Build history of the part. All positions in model axes, mm. Face numbers are marked on the shaded views. A direction names the side the tool comes from. Round coordinates to 2 decimals unless told otherwise and drop trailing zeros. Loops run counter-clockwise (first coordinate to the right, second up) from the corner with the lowest first, then second, coordinate; pieces in that order, holes last. Notation, with made-up numbers: (-26.5, 18.25) -> (19.5, 18.25) arc R33 cw to (19.5, 56.25) -> close; hole circle Ø11 at (-19.75, 26.5). An arc over 180 degrees is marked (long way). Put each result on its own line as item: value. Start each with the question number.
Item 1: Drill centre lines: probe 1 along Y at (x, z) = (67, 1); probe 2 along Z at (x, y) = (21, 14.5); probe 3 along Y at (x, z) = (-8, -48.5). Where is each one in solid material? Low to high. Write a range as [from, to].
Item 2: Flat gauge pins, fed straight in: pin 1 Ø5 at (y, z) = (3, -14.5) entering from +X; pin 2 Ø2 at (x, y) = (67, 36) entering from -Z; pin 3 Ø0.6 at (x, y) = (-4.5, -7.5) entering from -Z; pin 4 Ø4 at (x, z) = (51.5, -25.5) entering from -Y. Where does each tip first touch, or does it go through?
Item 3: Cut at D-D, the plane y = 36. List the corners of the cut face in (x, z), plus the area to 3 significant figures.
Item 4: Cut at C-C, the plane z = -14. List the corners of the cut face in (x, y), plus the area to 3 significant figures.
Item 5: Cut at A-A, the plane y = 0. List the corners of the cut face in (x, z) (3 decimals), plus the area to 3 significant figures.
Item 6: Cut at B-B, the plane x = 67. List the corners of the cut face in (y, z), plus the area to 3 significant figures.
Item 7: Tool access for the marked faces 1 and 2: list every direction of +Z, -Z, +X, -X, +Y, -Y with a clear straight run to the whole face (end or side of a thin tool).
Item 8: Pull direction Z, two halves, no side cores. Call the marked faces 3, 4 and 5: +Z half, -Z half, draft (parallel to the pull), parting line (faces both ways), or undercut.
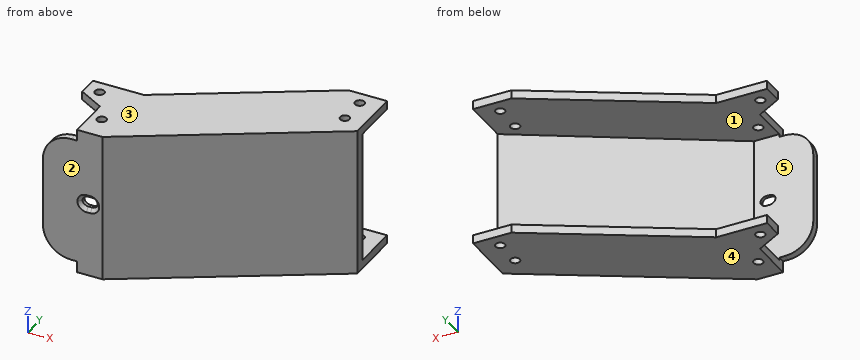
```python
from build123d import *

# Parameters (mm, degrees)
SKETCH1_R                                      = 1.65
BOSS_EXTRUDE1_DEPTH                            = 3
SKETCH1_3_W                                    = 9
SKETCH1_3_H                                    = 2.5
BOSS_EXTRUDE2_DEPTH                            = 46.6
BOSS_EXTRUDE3_START                            = -49.6
SKETCH1_4_R                                    = 1.65
SKETCH1_4_W                                    = 9
SKETCH1_4_H                                    = 2.5
BOSS_EXTRUDE3_DEPTH                            = 3
CUT_EXTRUDE1_DEPTH                             = 88.5
SKETCH3_W                                      = 44.6
SKETCH3_H                                      = 2.5
BOSS_EXTRUDE4_DEPTH                            = 12
FILLET1_R                                      = 10
CSK_START                                      = -9
CSK_SLOT_FOR_M3_COUNTERSUNK_FLAT_HEAD_SC_DEPTH = 3


with BuildPart() as part:
    # Sketch1 → Boss-Extrude1 (new body)
    with BuildSketch(Plane.XY):
        Polygon((-13, 18.856406461), (-13, 11.696152423), (-4, 6.5), (-4, -9), (5, -9), (74, 31), (74, 51), (60.447698856, 51), (5, 18.856406461), align=None)
        Circle(SKETCH1_R, mode=Mode.SUBTRACT)
        with Locations((-8, 13.856406461)):
            Circle(SKETCH1_R, mode=Mode.SUBTRACT)
        with Locations((67, 46)):
            Circle(SKETCH1_R, mode=Mode.SUBTRACT)
        with Locations((67, 36)):
            Circle(SKETCH1_R, mode=Mode.SUBTRACT)
    extrude(amount=BOSS_EXTRUDE1_DEPTH)

    # Sketch1<3> → Boss-Extrude2 (add)
    with BuildSketch(Plane.XY):
        with Locations((0.5, -7.75)):
            Rectangle(SKETCH1_3_W, SKETCH1_3_H)
        Polygon((74, 34.467646849), (5, -6.5), (5, -9), (74, 31), align=None)
    extrude(amount=-BOSS_EXTRUDE2_DEPTH)

    # Sketch1<4> → Boss-Extrude3 (add)
    # profile 1 of 4: a face of its own
    with BuildSketch(Plane.XY.offset(BOSS_EXTRUDE3_START)):
        Polygon((5, 18.856406461), (-13, 18.856406461), (-13, 11.696152423), (-4, 6.5), (-4, -6.5), (5, -6.5), align=None)
        Circle(SKETCH1_4_R, mode=Mode.SUBTRACT)
        with Locations((-8, 13.856406461)):
            Circle(SKETCH1_4_R, mode=Mode.SUBTRACT)
    # profile 2 of 4: a face of its own
    with BuildSketch(Plane.XY.offset(BOSS_EXTRUDE3_START)):
        with Locations((0.5, -7.75)):
            Rectangle(SKETCH1_4_W, SKETCH1_4_H)
    # profile 3 of 4: a face of its own
    with BuildSketch(Plane.XY.offset(BOSS_EXTRUDE3_START)):
        Polygon((74, 34.467646849), (5, -6.5), (5, -9), (74, 31), align=None)
    # profile 4 of 4: a face of its own
    with BuildSketch(Plane.XY.offset(BOSS_EXTRUDE3_START)):
        Polygon((60.447698856, 51), (5, 18.856406461), (5, -6.5), (74, 34.467646849), (74, 51), align=None)
        with Locations((67, 36)):
            Circle(SKETCH1_4_R, mode=Mode.SUBTRACT)
        with Locations((67, 46)):
            Circle(SKETCH1_4_R, mode=Mode.SUBTRACT)
    extrude(amount=BOSS_EXTRUDE3_DEPTH)

    # Sketch2 → Cut-Extrude1 (cut)
    with BuildSketch(Plane.XZ.offset(9)):
        with BuildLine():
            Line((1, -24.95), (-1, -24.95))
            ThreePointArc((-1, -24.95), (-2.65, -23.3), (-1, -21.65))
            Line((-1, -21.65), (1, -21.65))
            ThreePointArc((1, -21.65), (2.65, -23.3), (1, -24.95))
        make_face()
    extrude(amount=-CUT_EXTRUDE1_DEPTH, mode=Mode.SUBTRACT)

    # Sketch3 → Boss-Extrude4 (add)
    with BuildSketch(Plane.ZY.offset(4)):
        with Locations((-23.3, -7.75)):
            Rectangle(SKETCH3_W, SKETCH3_H)
    extrude(amount=BOSS_EXTRUDE4_DEPTH)

    # Fillet1
    fillet1_edges = [part.edges().sort_by_distance(p)[0] for p in [
        (-16, -7.75, -45.6),
        (-16, -7.75, -1),
    ]]
    fillet(fillet1_edges, radius=FILLET1_R)

    # CSK SLOT for M3 Countersunk Flat Head Screw1: read off the stored shape, not the designer's step
    # CSK SLOT for M3 Countersunk Flat Hea 2 → CSK SLOT for M3 Countersunk Flat Head Screw1 (cut)
    with BuildSketch(Plane(origin=(0, 0, 0), x_dir=(1, 0, 0), z_dir=(0, 1, 0)).offset(CSK_START)):
        with BuildLine():
            ThreePointArc((-1.7125, 21.811764888), (-1.229705955, 21.579705955), (-0.7, 21.5))
            Line((-0.7, 21.5), (0.7, 21.5))
            ThreePointArc((0.7, 21.5), (1.229705955, 21.579705955), (1.7125, 21.811764888))
            ThreePointArc((1.7125, 21.811764888), (1.365316345, 21.690949358), (1, 21.65))
            Line((1, 21.65), (-1, 21.65))
            ThreePointArc((-1, 21.65), (-1.365316345, 21.690949358), (-1.7125, 21.811764888))
        make_face()
        with BuildLine():
            ThreePointArc((-0.7, 25.1), (-1.229705955, 25.020294045), (-1.7125, 24.788235112))
            ThreePointArc((-1.7125, 24.788235112), (-1.365316345, 24.909050642), (-1, 24.95))
            Line((-1, 24.95), (1, 24.95))
            ThreePointArc((1, 24.95), (1.365316345, 24.909050642), (1.7125, 24.788235112))
            ThreePointArc((1.7125, 24.788235112), (1.229705955, 25.020294045), (0.7, 25.1))
            Line((0.7, 25.1), (-0.7, 25.1))
        make_face()
    extrude(amount=CSK_SLOT_FOR_M3_COUNTERSUNK_FLAT_HEAD_SC_DEPTH, mode=Mode.SUBTRACT)

    # CSK SLOT for M3 Countersunk Flat Hea 3: loft between two sections, ruled curve by curve
    csk_slot_for_m3_countersunk_flat_hea_3_from = [
        Edge.make_three_point_arc((0.7, -7.649999999, -25.099999999), (1.972792205, -7.649999999, -24.572792205), (2.499999999, -7.649999999, -23.3)),
        Edge.make_three_point_arc((2.499999999, -7.649999999, -23.3), (1.972792205, -7.649999999, -22.027207795), (0.7, -7.649999999, -21.500000001)),
        Edge.make_three_point_arc((-0.7, -7.649999999, -21.500000001), (-1.972792205, -7.649999999, -22.027207795), (-2.499999999, -7.649999999, -23.3)),
        Edge.make_three_point_arc((-2.499999999, -7.649999999, -23.3), (-1.972792205, -7.649999999, -24.572792205), (-0.7, -7.649999999, -25.099999999)),
        Edge.make_line((0.7, -7.649999999, -21.500000001), (-0.7, -7.649999999, -21.500000001)),
        Edge.make_line((0.7, -7.649999999, -25.099999999), (-0.7, -7.649999999, -25.099999999)),
    ]
    csk_slot_for_m3_countersunk_flat_hea_3_to = [
        Edge.make_three_point_arc((0.7, -9, -26.45), (2.927386361, -9, -25.527386361), (3.85, -9, -23.3)),
        Edge.make_three_point_arc((3.85, -9, -23.3), (2.927386361, -9, -21.072613639), (0.7, -9, -20.15)),
        Edge.make_three_point_arc((-0.7, -9, -20.15), (-2.927386361, -9, -21.072613639), (-3.85, -9, -23.3)),
        Edge.make_three_point_arc((-3.85, -9, -23.3), (-2.927386361, -9, -25.527386361), (-0.7, -9, -26.45)),
        Edge.make_line((0.7, -9, -20.15), (-0.7, -9, -20.15)),
        Edge.make_line((0.7, -9, -26.45), (-0.7, -9, -26.45)),
    ]
    csk_slot_for_m3_countersunk_flat_hea_3 = Solid(Shell([*[Face.make_surface_from_curves(csk_slot_for_m3_countersunk_flat_hea_3_from[k], csk_slot_for_m3_countersunk_flat_hea_3_to[k]) for k in range(6)], Face(Wire(csk_slot_for_m3_countersunk_flat_hea_3_from)), Face(Wire(csk_slot_for_m3_countersunk_flat_hea_3_to))]))
    add(csk_slot_for_m3_countersunk_flat_hea_3, mode=Mode.SUBTRACT)


solid = part.part
```
Reply:
1. probe 1: y = [26.94, 34.35], [37.65, 44.35], [47.65, 51]
1. probe 2: z = [-49.6, -46.6], [0, 3]
1. probe 3: y = [8.81, 12.21], [15.51, 18.86]
2. pin 1: stops at x = 30.01
2. pin 2: passes through
2. pin 3: stops at z = -45.6
2. pin 4: stops at y = 16.8
3. outline: (34.57, -49.6) -> (65.35, -49.6) -> (65.35, -46.6) -> (34.57, -46.6) -> close; (34.57, 0) -> (65.35, 0) -> (65.35, 3) -> (34.57, 3) -> close; (68.65, -49.6) -> (74, -49.6) -> (74, -46.6) -> (68.65, -46.6) -> close; (68.65, 0) -> (74, 0) -> (74, 3) -> (68.65, 3) -> close
3. area: 217 mm^2
4. outline: (-16, -9) -> (5, -9) -> (74, 31) -> (74, 34.47) -> (5, -6.5) -> (-16, -6.5) -> close
4. area: 258 mm^2
5. outline: (-4, -49.6) -> (-1.65, -49.6) -> (-1.65, -46.6) -> (-4, -46.6) -> close; (-4, 0) -> (-1.65, 0) -> (-1.65, 3) -> (-4, 3) -> close; (1.65, -49.6) -> (20.525, -49.6) -> (20.525, 3) -> (1.65, 3) -> (1.65, 0) -> (15.948, 0) -> (15.948, -46.6) -> (1.65, -46.6) -> close
5. area: 341 mm^2
6. outline: (26.94, -49.6) -> (34.35, -49.6) -> (34.35, -46.6) -> (30.31, -46.6) -> (30.31, 0) -> (34.35, 0) -> (34.35, 3) -> (26.94, 3) -> close; (37.65, -49.6) -> (44.35, -49.6) -> (44.35, -46.6) -> (37.65, -46.6) -> close; (37.65, 0) -> (44.35, 0) -> (44.35, 3) -> (37.65, 3) -> close; (47.65, -49.6) -> (51, -49.6) -> (51, -46.6) -> (47.65, -46.6) -> close; (47.65, 0) -> (51, 0) -> (51, 3) -> (47.65, 3) -> close
6. area: 262 mm^2
7. face 1: -X, +Y
7. face 2: +Z, -Z, +X, -X, -Y
8. face 3: +Z half
8. face 4: -Z half
8. face 5: undercut
